```python
from build123d import *

# Parameters (mm, degrees)
SKETCH_1_R          = 7.5
EXTRUDE_1_DEPTH     = 87.5
SKETCH_2_W          = 10
SKETCH_2_H          = 15
EXTRUDE_2_DEPTH     = 7.5
SKETCH_3_R          = 4
EXTRUDE_3_DEPTH     = 15
SKETCH_4_W          = 10
SKETCH_4_H          = 15
EXTRUDE_4_DEPTH     = 7.5
SKETCH_5_R          = 4
CUT_EXTRUDE_1_DEPTH = 15
FILLET_1_R          = 3


with BuildPart() as part:
    # 草图1 → 凸台-拉伸1 (new, symmetric)
    with BuildSketch(Plane.XY):
        Circle(SKETCH_1_R)
    extrude(amount=EXTRUDE_1_DEPTH, both=True)

    # 草图2 → 凸台-拉伸2 (add)
    with BuildSketch(Plane(origin=(0, 0, 0), x_dir=(0, 0, -1), z_dir=(1, 0, 0))):
        with Locations((-82.5, 0)):
            Rectangle(SKETCH_2_W, SKETCH_2_H)
    extrude(amount=-EXTRUDE_2_DEPTH)

    # 草图3 → 凸台-拉伸3 (add)
    with BuildSketch(Plane.ZY.offset(7.5)):
        with Locations((82.5, 0)):
            Circle(SKETCH_3_R)
    extrude(amount=EXTRUDE_3_DEPTH)

    # 草图4 → 凸台-拉伸4 (add)
    with BuildSketch(Plane(origin=(0, 0, 0), x_dir=(0, 0, -1), z_dir=(1, 0, 0))):
        with Locations((82.5, 0)):
            Rectangle(SKETCH_4_W, SKETCH_4_H)
    extrude(amount=EXTRUDE_4_DEPTH)

    # 草图5 → 切除-拉伸1 (cut)
    with BuildSketch(Plane(origin=(7.5, 0, 0), x_dir=(0, 0, -1), z_dir=(1, 0, 0))):
        with Locations((82.5, 0)):
            Circle(SKETCH_5_R)
    extrude(amount=-CUT_EXTRUDE_1_DEPTH, mode=Mode.SUBTRACT)

    # 圆角1
    fillet_1_edges = [part.edges().sort_by_distance(p)[0] for p in [
        (-3.75, -7.5, 87.5),
        (-7.5, 7.5, 82.5),
        (-3.75, 7.5, 87.5),
        (-7.5, -7.5, 82.5),
        (5.303300859, -5.303300859, 87.5),
    ]]
    fillet(fillet_1_edges, radius=FILLET_1_R)


solid = part.part
```
Here's how the part is built. I have some questions about the finished solid (model axes, mm). A direction names the side the tool comes from. Round coordinates to 2 decimals unless told otherwise and drop trailing zeros. Write each loop counter-clockwise with the first axis right and the second up, starting at its lowest first coordinate (ties: lowest second). Pieces come first, ordered by that corner, then holes.
Q1. Please list where these lines run through material, in increasing order: probe 1 along Z at (x, y) = (-2.5, 0); probe 2 along Y at (x, z) = (2, -82.5); probe 3 along Z at (x, y) = (-5, -4.75).
Q2. If we mould it in two halves opening along Y, with no side actions, what happens to faces 5 (the cylindrical face through (0.105, -1.532, -86.195)), 6 (the flat face through (7.5, 0, -78)), 7 (the cylindrical face through (-14.895, 0.176, 78.504)), 8 (the flat face through (4, 7.5, -82))? For each: +Y half, -Y half, draft (parallel to the pull), parting line (faces both ways), or undercut.
Q3. If we section it at A-A on z = -82.5: Write out the boundary of the cut face in (x, y).
Q4. If we section it at D-D on z = 53: Write out the boundary of the cut face in (x, y).
Q5. Will these pins go through, and if not, where does the flat tip stop? P1, Ø1.5, axis at y = -5.5, z = -22, coming from the -X side; P2, Ø1.5, axis at x = 4, z = 37, coming from the +Y side; P3, Ø6, axis at x = -13.5, y = 5.5, coming from the +Z side; P4, Ø6, axis at x = 5, y = 2.5, coming from the +Z side.
Q6. Which directions (+Z, -Z, +X, -X, +Y, -Y) give clear straight access to the entire face, cutting with the end or side of a thin tool? Please do faces 1 (the flat face through (-6, -6, 77.5)), 2 (the flat face through (-6, 6, 77.5)), 3 (the flat face through (6, -6, -77.5)), 4 (the cylindrical face through (-7.493, 0.33, -0.296)).
Q7. If we section it at B-B on z = 82.5: Write out the boundary of the cut face in (x, y), plus the area to 3 significant figures.
Q8. If we section it at C-C on x = -14: Write out the boundary of the cut face in (y, z).
Answer below:
1. probe 1: z = -87.5 to -86.5, -78.5 to 87.5
1. probe 2: y = -7.5 to -4, 4 to 7.5
1. probe 3: z = -87.5 to 87.49
2. face 5: undercut
2. face 6: draft
2. face 7: parting line
2. face 8: +Y half
3. outline: (-6.34, -4) arc R7.5 ccw to (0, -7.5) - (7.5, -7.5) - (7.5, -4) - close; (-6.34, 4) - (7.5, 4) - (7.5, 7.5) - (0, 7.5) arc R7.5 ccw to start
4. outline: circle Ø15 at (0, 0)
5. P1: stops at x = -5.8
5. P2: stops at y = 6.76
5. P3: stops at z = 85.62
5. P4: stops at z = 87.5
6. face 1: -Z, -X, -Y
6. face 2: -Z, -X, +Y
6. face 3: +Z, +X, -Y
6. face 4: none
7. outline: (-22.5, -4) - (-7.5, -4) - (-7.5, -4.5) arc R3 ccw to (-4.5, -7.5) - (0, -7.5) arc R7.5 ccw to (0, 7.5) - (-4.5, 7.5) arc R3 ccw to (-7.5, 4.5) - (-7.5, 4) - (-22.5, 4) - close
7. area: 317 mm2
8. outline: circle Ø8 at (0, 82.5)
